Input: part model. Units: mm. Frame: model coordinates. Round coordinates to 2 decimals unless told otherwise and drop trailing zeros. Loops run counter-clockwise (first coordinate to the right, second up) from the corner with the lowest first, then second, coordinate; pieces in that order, holes last. Notation, with made-up numbers: (-9.75, 37) - (5.25, 37) arc R20 ccw to (5.25, 67) - close; hole circle Ø3 at (84.5, 68.25). An arc over 180 degrees is marked (long way). Use CSV: the item, a comma, the result in double quotes. Start each with the question number.
1. Cut plane C-C (x = 8.5). Return loops of the section in (y, z), and give its area (3 significant figures).
2. Cut plane A-A (x = 0). Return loops of the section in (y, z).
3. Pin query (flat end, axial travel): P1, Ø17, axis at x = 0, y = 0, coming from the -Z side; P2, Ø6, axis at x = 16, y = -12.5, coming from the +Z side. Return the tip coordinate at first contact, or that it passes through.
4. Cut plane B-B (y = -13). Return loops of the section in (x, z).
5. Material intervals for probe 1 along Y at (x, z) = (0, -0.9); probe 2 along X at (y, z) = (1, -0.6); probe 3 along X at (y, z) = (-0.5, -0.4), sorted ascending. Write a range as from..to.
```python
from build123d import *

# Parameters (mm, degrees)
SKETCH1_R          = 26.9875
SKETCH1_R_2        = 14.2875
BASE_FLANGE1_DEPTH = 1.5875
SKETCH6_R          = 1.651
CUT_EXTRUDE1_DEPTH = 39.199089894


# Sheet-metal steps are written as plain solids
with BuildPart() as part:
    # Sketch1 → Base-Flange1 (new body)
    with BuildSketch(Plane.XY):
        Circle(SKETCH1_R)
        Circle(SKETCH1_R_2, mode=Mode.SUBTRACT)
    extrude(amount=-BASE_FLANGE1_DEPTH)

    # Sketch6 → Cut-Extrude1 (cut, through all)
    with BuildSketch(Plane.XY):
        with Locations((0, 20.6375)):
            Circle(SKETCH6_R)
        with Locations((20.6375, 0)):
            Circle(SKETCH6_R)
        with Locations((0, -20.6375)):
            Circle(SKETCH6_R)
        with Locations((-20.6375, 0)):
            Circle(SKETCH6_R)
    extrude(amount=-CUT_EXTRUDE1_DEPTH, mode=Mode.SUBTRACT)


solid = part.part
```
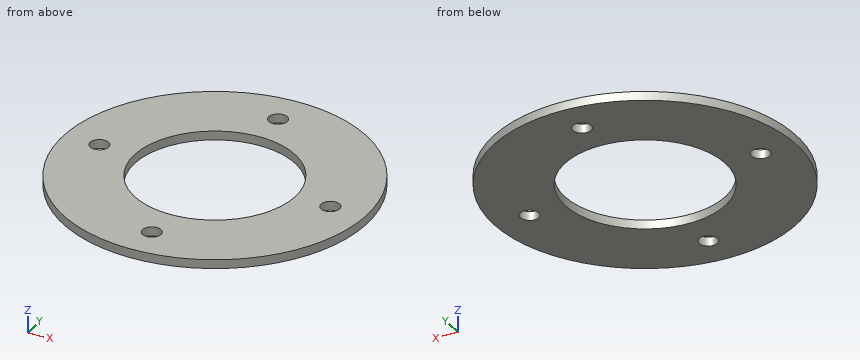
Established:
1,outline,"(-25.61, -1.59) - (-11.48, -1.59) - (-11.48, 0) - (-25.61, 0) - close; (11.48, -1.59) - (25.61, -1.59) - (25.61, 0) - (11.48, 0) - close"
1,area,"44.9 mm2"
2,outline,"(-26.99, -1.59) - (-22.29, -1.59) - (-22.29, 0) - (-26.99, 0) - close; (-18.99, -1.59) - (-14.29, -1.59) - (-14.29, 0) - (-18.99, 0) - close; (14.29, -1.59) - (18.99, -1.59) - (18.99, 0) - (14.29, 0) - close; (22.29, -1.59) - (26.99, -1.59) - (26.99, 0) - (22.29, 0) - close"
3,P1,"passes through"
3,P2,"stops at z = 0"
4,outline,"(-23.65, -1.59) - (-5.93, -1.59) - (-5.93, 0) - (-23.65, 0) - close; (5.93, -1.59) - (23.65, -1.59) - (23.65, 0) - (5.93, 0) - close"
5,probe 1,"y = -26.99..-22.29, -18.99..-14.29, 14.29..18.99, 22.29..26.99"
5,probe 2,"x = -26.97..-21.95, -19.32..-14.25, 14.25..19.32, 21.95..26.97"
5,probe 3,"x = -26.98..-22.21, -19.06..-14.28, 14.28..19.06, 22.21..26.98"
